The model under review builds one solid part; all positions refer to its coordinate system, in mm. Round coordinates to 2 decimals unless told otherwise and drop trailing zeros. Loops run counter-clockwise (first coordinate to the right, second up) from the corner with the lowest first, then second, coordinate; pieces in that order, holes last. Notation, with made-up numbers: M 3,-18 L 57,-18 A15 cw 57,0 Z; hole C 84,-15.75 d2. An arc over 180 degrees is marked long. Return JSON: item names as keys, results as strings. Group by question number.
Q1. Consider section D-D (y = -0.75). State the section outline as (x, z) points, and give its area (3 significant figures).
Q2. Consider section A-A (y = 0). State the section outline as (x, z) points, and give its area (3 significant figures).
Q3. Consider section B-B (x = -5). State the section outline as (y, z) points, and give its area (3 significant figures).
Q4. Consider section C-C (z = -0.1). State the section outline as (x, y) points.
Q5. To check wall thickness, follow line 1 along X through (y, z) = (0.1, -0.2); line 2 along Y through (x, z) = (-5, -0.05); line 3 along Y through (x, z) = (-0.25, -0.05). State the ranges of each line that lie inside material, in increasing order.
from build123d import *

# Parameters (mm, degrees)
F0_R     = 0.5
F1_DEPTH = 0.25


with BuildPart() as f1:
    # F0 (on Top) → F1 (new body, symmetric)
    with BuildSketch(Plane.XY):
        with BuildLine():
            Line((-7, 1.25), (-7, 0))
            Line((-7, 0), (-7, -1.25))
            Line((-7, -1.25), (-4, -1.25))
            ThreePointArc((-4, -1.25), (-2.0615528128, -0.5037887488), (0, -0.25))
            ThreePointArc((0, -0.25), (2.0615528128, -0.5037887488), (4, -1.25))
            Line((4, -1.25), (7, -1.25))
            Line((7, -1.25), (7, 0))
            Line((7, 0), (7, 1.25))
            Line((7, 1.25), (4, 1.25))
            ThreePointArc((4, 1.25), (2.0615528128, 0.5037887488), (0, 0.25))
            ThreePointArc((0, 0.25), (-2.0615528128, 0.5037887488), (-4, 1.25))
            Line((-4, 1.25), (-7, 1.25))
        make_face()
        with Locations((-5, 0)):
            Circle(F0_R, mode=Mode.SUBTRACT)
        with Locations((5, 0)):
            Circle(F0_R, mode=Mode.SUBTRACT)
    extrude(amount=F1_DEPTH, both=True)


solid = f1.part
Values:
{
 "1": {"outline": "M -7,-0.25 L -2.87,-0.25 L -2.87,0.25 L -7,0.25 Z; M 2.87,-0.25 L 7,-0.25 L 7,0.25 L 2.87,0.25 Z", "area": "4.13 mm2"},
 "2": {"outline": "M -7,-0.25 L -5.5,-0.25 L -5.5,0.25 L -7,0.25 Z; M -4.5,-0.25 L 4.5,-0.25 L 4.5,0.25 L -4.5,0.25 Z; M 5.5,-0.25 L 7,-0.25 L 7,0.25 L 5.5,0.25 Z", "area": "6.00 mm2"},
 "3": {"outline": "M -1.25,-0.25 L -0.5,-0.25 L -0.5,0.25 L -1.25,0.25 Z; M 0.5,-0.25 L 1.25,-0.25 L 1.25,0.25 L 0.5,0.25 Z", "area": "0.750 mm2"},
 "4": {"outline": "M -7,-1.25 L -4,-1.25 A8.5 cw 4,-1.25 L 7,-1.25 L 7,1.25 L 4,1.25 A8.5 cw -4,1.25 L -7,1.25 Z; hole C -5,0 d1; hole C 5,0 d1"},
 "5": {"line 1": "x = -7 to -5.49, -4.51 to 4.51, 5.49 to 7", "line 2": "y = -1.25 to -0.5, 0.5 to 1.25", "line 3": "y = -0.25 to 0.25"}
}
